Check sheet for the drawn part. Datum: minimum x, y, z corner. Units: mm. Round coordinates to 2 decimals unless told otherwise and drop trailing zeros. Write each loop counter-clockwise with the first axis right and the second up, starting at its lowest first coordinate (ties: lowest second). Pieces come first, ordered by that corner, then holes. Notation, with made-up numbers: M 89.5,-9.75 L 107.5,-9.75 A17 cw 107.5,17.25 Z; hole C 85,-12 d8. An arc over 180 degrees is marked long. One line per item, written item: value. Start each with the question number.
1. Section check A-A (z = 1.3). Record the boundary of the cut face in (x, y) (3 decimals).
2. Depth check by flat-ended pin: P1, Ø1.6, axis at y = 27.5, z = 2, coming from the +X side (3 decimals); P2, Ø1.6, axis at x = 24.5, z = 1.5, coming from the -Y side; P3, Ø1.6, axis at x = 20.5, z = 1, coming from the +Y side (3 decimals). Enter the tip coordinate at first touch or a pass-through.
3. Scan lines: probe 1 along Y at (x, z) = (23.75, 2.75); probe 2 along X at (y, z) = (46, 1.45) (3 decimals); probe 3 along Y at (x, z) = (9.25, 1.3) (3 decimals). Record each from-to range of solid material in increasing order. Write a range as [from, to].
4. Section check B-B (x = 13.5). Record the boundary of the cut face in (y, z) (3 decimals).
5. Section check C-C (y = 53.5). Record the boundary of the cut face in (x, z) (3 decimals).
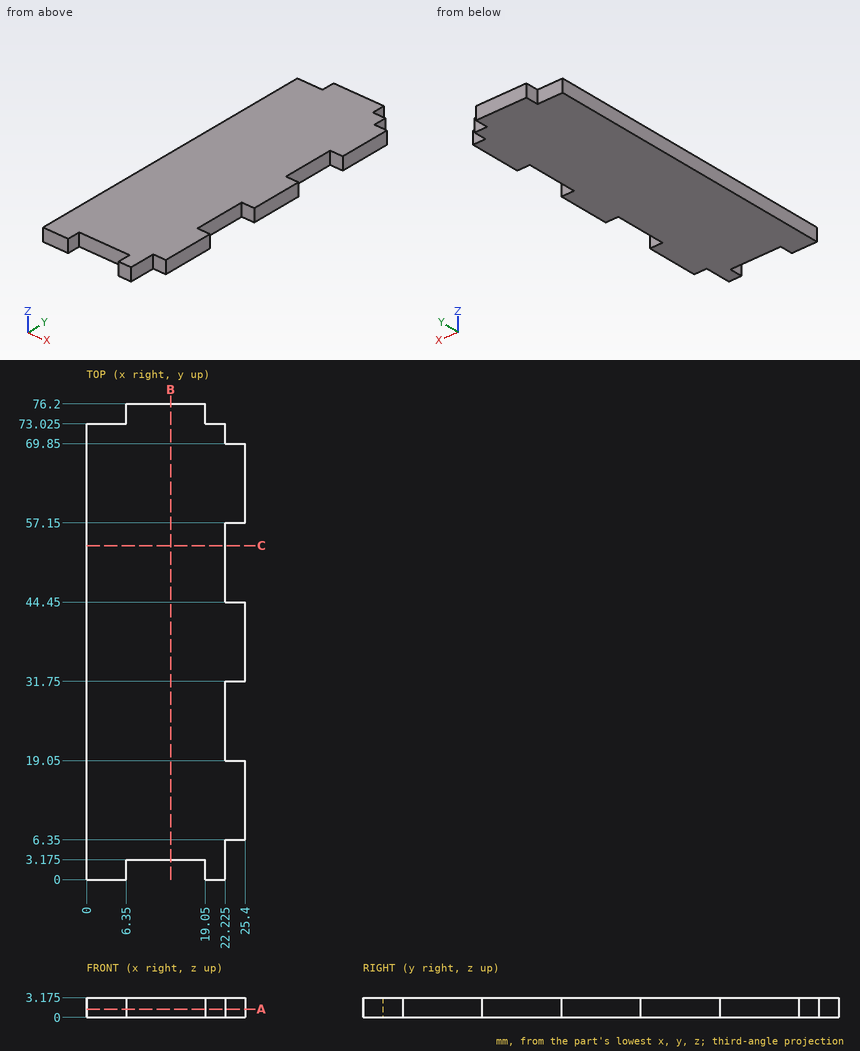
Result sheet:
1. outline: M 0,0 L 6.35,0 L 6.35,3.175 L 19.05,3.175 L 19.05,0 L 22.225,0 L 22.225,6.35 L 25.4,6.35 L 25.4,19.05 L 22.225,19.05 L 22.225,31.75 L 25.4,31.75 L 25.4,44.45 L 22.225,44.45 L 22.225,57.15 L 25.4,57.15 L 25.4,69.85 L 22.225,69.85 L 22.225,73.025 L 19.05,73.025 L 19.05,76.2 L 6.35,76.2 L 6.35,73.025 L 0,73.025 Z
2. P1: stops at x = 22.225
2. P2: stops at y = 6.35
2. P3: stops at y = 73.025
3. probe 1: y = [6.35, 19.05], [31.75, 44.45], [57.15, 69.85]
3. probe 2: x = [0, 22.225]
3. probe 3: y = [3.175, 76.2]
4. outline: M 3.175,0 L 76.2,0 L 76.2,3.175 L 3.175,3.175 Z
5. outline: M 0,0 L 22.225,0 L 22.225,3.175 L 0,3.175 Z
